Part print with two shaded views. Sizes in mm from the minimum x, y, z corner. A direction names the side the tool comes from. Coordinates: 2 decimals unless noted, no trailing zeros. Loops run counter-clockwise (first coordinate to the right, second up) from the corner with the lowest first, then second, coordinate; pieces in that order, holes last. Notation, with made-up numbers: (-4, 36) -> (32, 36) arc R32 cw to (32, 75) -> close; hole circle Ø4 at (72.5, 56). An arc over 180 degrees is marked (long way). Write each question's results on one line, items separated by ' | '.
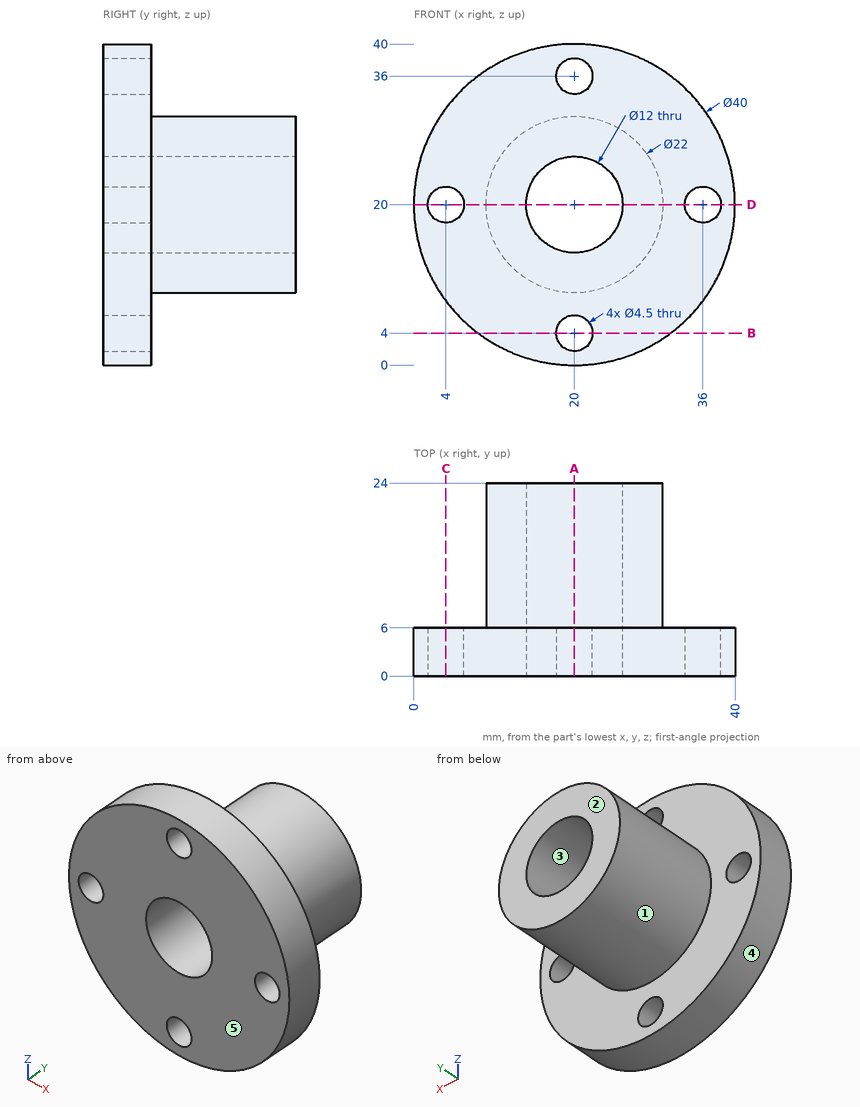
Q1. Cut at D-D on z = 20. Write the cut outline in (x, y).
Results are:
outline: (0, 0) -> (1.75, 0) -> (1.75, 6) -> (0, 6) -> close; (6.25, 0) -> (14, 0) -> (14, 24) -> (9, 24) -> (9, 6) -> (6.25, 6) -> close; (26, 0) -> (33.75, 0) -> (33.75, 6) -> (31, 6) -> (31, 24) -> (26, 24) -> close; (38.25, 0) -> (40, 0) -> (40, 6) -> (38.25, 6) -> close
Q2. Wall check: L1, parallel to Z at x = 20, y = 1.45; L2, parallel to Y at x = 30, z = 33; L3, parallel to X at y = 5.5, z = 35. Give the ranges that are in metal, low to high. Write a range as from..to.
Results are:
L1: 0..1.75, 6.25..14, 26..33.75, 38.25..40 | L2: 0..6 | L3: 6.77..17.98, 22.02..33.23
Q3. Pull direction Z, two halves, no side cores. Call the marked faces 3, 4 and 5: +Z half, -Z half, draft (parallel to the pull), parting line (faces both ways), or undercut.
Results are:
face 3: undercut | face 4: parting line | face 5: draft
Q4. Cut at A-A on x = 20. Write the cut outline in (y, z), and give its area (3 significant figures).
Results are:
outline: (0, 0) -> (6, 0) -> (6, 1.75) -> (0, 1.75) -> close; (0, 6.25) -> (6, 6.25) -> (6, 9) -> (24, 9) -> (24, 14) -> (0, 14) -> close; (0, 26) -> (24, 26) -> (24, 31) -> (6, 31) -> (6, 33.75) -> (0, 33.75) -> close; (0, 38.25) -> (6, 38.25) -> (6, 40) -> (0, 40) -> close | area: 294 mm^2
Q5. Which spindle directions (+Z, -Z, +X, -X, +Y, -Y) get a long thin tool onto all of the face, cutting with end or side? Do the marked faces 1 and 2. Say none if no direction does.
Results are:
face 1: +Y | face 2: +Z, -Z, +X, -X, +Y
Q6. Cut at B-B on z = 4. Write the cut outline in (x, y).
Results are:
outline: (8, 0) -> (17.75, 0) -> (17.75, 6) -> (8, 6) -> close; (22.25, 0) -> (32, 0) -> (32, 6) -> (22.25, 6) -> close
Q7. Cut at C-C on x = 4. Write the cut outline in (y, z).
Results are:
outline: (0, 8) -> (6, 8) -> (6, 17.75) -> (0, 17.75) -> close; (0, 22.25) -> (6, 22.25) -> (6, 32) -> (0, 32) -> close
Q8. Drop flat-ended pins along their axis: pin 1 (4 mm diameter, centred on x = 36, z = 20, fed in from -Y); pin 2 (2 mm diameter, centred on x = 6.5, z = 8.5, fed in from +Y); pin 3 (3 mm diameter, centred on y = 20, z = 17, fed in from -X); pin 4 (2 mm diameter, centred on y = 4.5, z = 35, fed in from -X). Give the stop position or say it passes through.
Results are:
pin 1: through | pin 2: y = 6 | pin 3: x = 9.1 | pin 4: x = 5.72
